from build123d import *

# Parameters (mm, degrees)
SKETCH_1_W          = 122
SKETCH_1_H          = 60
SKETCH_1_R          = 7
SKETCH_1_R_2        = 2.1
EXTRUDE_1_DEPTH     = 2.45
FILLET_1_R          = 9
SKETCH_2_W          = 2.45
SKETCH_2_H          = 60
EXTRUDE_2_DEPTH     = 61
FILLET_2_R          = 4
CUT_EXTRUDE_1_DEPTH = 61


with BuildPart() as part:
    # 草图1 → 凸台-拉伸1 (new body)
    with BuildSketch(Plane(origin=(0, 0, 0), x_dir=(1, 0, 0), z_dir=(0, 1, 0))):
        Rectangle(SKETCH_1_W, SKETCH_1_H)
        with Locations(Location((-41.45, 0, 0), (0, 0, 270))):
            Circle(SKETCH_1_R, mode=Mode.SUBTRACT)
        with Locations(Location((-41.45, 20, 0), (0, 0, 270))):
            Circle(SKETCH_1_R_2, mode=Mode.SUBTRACT)
        with Locations(Location((-1.45, 20, 0), (0, 0, 270))):
            Circle(SKETCH_1_R_2, mode=Mode.SUBTRACT)
        with Locations(Location((-1.45, -20, 0), (0, 0, 270))):
            Circle(SKETCH_1_R_2, mode=Mode.SUBTRACT)
        with Locations(Location((-41.45, -20, 0), (0, 0, 270))):
            Circle(SKETCH_1_R_2, mode=Mode.SUBTRACT)
    extrude(amount=EXTRUDE_1_DEPTH)

    # 圆角1
    fillet_1_edges = [part.edges().sort_by_distance(p)[0] for p in [
        (-61, 1.225, -30),
        (-61, 1.225, 30),
    ]]
    fillet(fillet_1_edges, radius=FILLET_1_R)

    # 草图2 → 凸台-拉伸2 (add)
    with BuildSketch(Plane(origin=(0, 2.45, 0), x_dir=(1, 0, 0), z_dir=(0, 1, 0))):
        with Locations((59.775, 0)):
            Rectangle(SKETCH_2_W, SKETCH_2_H)
    extrude(amount=EXTRUDE_2_DEPTH)

    # 圆角2
    fillet_2_edges = [part.edges().sort_by_distance(p)[0] for p in [
        (59.775, 63.45, -30),
        (59.775, 63.45, 30),
    ]]
    fillet(fillet_2_edges, radius=FILLET_2_R)

    # 草图3 → 切除-拉伸1 (cut)
    with BuildSketch(Plane.ZY.offset(-58.55)):
        with BuildLine():
            Line((-20.5, 47.5), (-20.5, 17))
            ThreePointArc((-20.5, 17), (-19, 15.5), (-17.5, 17))
            Line((-17.5, 17), (-17.5, 47.5))
            ThreePointArc((-17.5, 47.5), (-19, 49), (-20.5, 47.5))
        make_face()
        with BuildLine():
            Line((17.5, 47.5), (17.5, 17))
            ThreePointArc((17.5, 17), (19, 15.5), (20.5, 17))
            Line((20.5, 17), (20.5, 47.5))
            ThreePointArc((20.5, 47.5), (19, 49), (17.5, 47.5))
        make_face()
    extrude(amount=-CUT_EXTRUDE_1_DEPTH, mode=Mode.SUBTRACT)


solid = part.part
The listing builds one solid part. Answer for the finished solid, in the listing's coordinates (mm). A direction names the side the tool comes from. Round coordinates to 2 decimals unless told otherwise and drop trailing zeros. Order: outer loops, then holes, each group sorted by start corner. A loop starts at its lowest first (then second) coordinate and runs counter-clockwise, first axis right, second up. Notation, with made-up numbers: (11, 38.5) -> (20, 38.5) arc R25 ccw to (20, 65.5) -> close; hole circle Ø8 at (9.25, 15.5). An arc over 180 degrees is marked (long way). One line per item, written item: value.
Item 1: For a pull along X with two mould halves and no side action, classify faces 4 (the cylindrical face through (-58.434, 1.242, -27.294)), 5 (the cylindrical face through (-34.51, 1.21, -0.91)), 6 (the flat face through (60, 32, -17.5)) as released by +X, released by -X, zero draft, split by the parting line, or undercut.
Taken from the geometry:
face 4: released by -X
face 5: undercut
face 6: zero draft
Item 2: Given P1, Ø3.5, axis at x = -41.45, z = 20, coming from the +Y side; P2, Ø10, axis at x = 18.5, z = 7.5, coming from the +Y side, each flat-ended and moving along its own axis, determine where each tip first touches the part or whether it passes through.
Taken from the geometry:
P1: passes through
P2: stops at y = 2.45
Item 3: Straight lines are drawn through the part: L1, parallel to X at y = 1.7, z = 20; L2, parallel to X at y = 1, z = 0; L3, parallel to X at y = 16, z = 16.5. For each, find the intervals that lie inside material, in ascending order.
Taken from the geometry:
L1: x = -61 to -43.55, -39.35 to -3.55, 0.65 to 61
L2: x = -61 to -48.45, -34.45 to 61
L3: x = 58.55 to 61
Item 4: Find section B-B, the plane y = 32. Give the vertices of the cut face in (x, z), then the cut area to 3 significant figures.
Taken from the geometry:
outline: (58.55, -30) -> (61, -30) -> (61, -20.5) -> (58.55, -20.5) -> close; (58.55, -17.5) -> (61, -17.5) -> (61, 17.5) -> (58.55, 17.5) -> close; (58.55, 20.5) -> (61, 20.5) -> (61, 30) -> (58.55, 30) -> close
area: 132 mm2
Item 5: Find section A-A, the plane x = -41.45. Give the vertices of the cut face in (y, z).
Taken from the geometry:
outline: (0, -30) -> (2.45, -30) -> (2.45, -22.1) -> (0, -22.1) -> close; (0, -17.9) -> (2.45, -17.9) -> (2.45, -7) -> (0, -7) -> close; (0, 7) -> (2.45, 7) -> (2.45, 17.9) -> (0, 17.9) -> close; (0, 22.1) -> (2.45, 22.1) -> (2.45, 30) -> (0, 30) -> close
Item 6: Find section D-D, the plane z = 3. Give the vertices of the cut face in (x, y), then the cut area to 3 significant figures.
Taken from the geometry:
outline: (-61, 0) -> (-47.77, 0) -> (-47.77, 2.45) -> (-61, 2.45) -> close; (-35.13, 0) -> (61, 0) -> (61, 63.45) -> (58.55, 63.45) -> (58.55, 2.45) -> (-35.13, 2.45) -> close
area: 417 mm2
Item 7: For faces 1 (the flat face through (58.55, 33, 0)), 2 (the cylindrical face through (-39.368, 1.208, -20.273)), 3 (the cylindrical face through (59.8, 15.5, 19)), determine the directions among +Z, -Z, +X, -X, +Y, -Y from which every point of the face is accessible in a straight line to the end or side of a thin tool.
Taken from the geometry:
face 1: +Z, -Z, -X, +Y
face 2: +Y, -Y
face 3: +X, -X
Item 8: Find section C-C, the plane x = -1.45. Give the vertices of the cut face in (y, z), then the cut area to 3 significant figures.
Taken from the geometry:
outline: (0, -30) -> (2.45, -30) -> (2.45, -22.1) -> (0, -22.1) -> close; (0, -17.9) -> (2.45, -17.9) -> (2.45, 17.9) -> (0, 17.9) -> close; (0, 22.1) -> (2.45, 22.1) -> (2.45, 30) -> (0, 30) -> close
area: 126 mm2
